Check sheet for the modelled part. Datum: model origin and axes. Units: mm. A direction names the side the tool comes from. Round coordinates to 2 decimals unless told otherwise and drop trailing zeros. Write each loop counter-clockwise with the first axis right and the second up, starting at its lowest first coordinate (ties: lowest second). Pieces come first, ordered by that corner, then holes. Notation, with made-up numbers: M -9.5,-39.75 L 2.5,-39.75 A19 ccw 2.5,-18.75 Z; hole C 52.25,17.25 d11. An arc over 180 degrees is marked long. Answer in a Markdown table with one row per item.
```python
from build123d import *

# Parameters (mm, degrees)
SKETCH1_W           = 45
SKETCH1_H           = 20
BOSS_EXTRUDE1_DEPTH = 1
SKETCH2_R           = 7.5
SKETCH2_R_2         = 6.5
BOSS_EXTRUDE2_DEPTH = 12
SKETCH3_R           = 6.5
BOSS_EXTRUDE3_DEPTH = 10


with BuildPart() as part:
    # Sketch1 → Boss-Extrude1 (new body)
    with BuildSketch(Plane.XY):
        with Locations((-3.47266881, 2.258842444)):
            Rectangle(SKETCH1_W, SKETCH1_H)
    extrude(amount=BOSS_EXTRUDE1_DEPTH)

    # Sketch2 → Boss-Extrude2 (add)
    with BuildSketch(Plane.XY):
        with Locations((-16.47266881, 2.258842444)):
            Circle(SKETCH2_R)
        with Locations((-16.47266881, 2.258842444)):
            Circle(SKETCH2_R_2, mode=Mode.SUBTRACT)
        with Locations((9.52733119, 2.258842444)):
            Circle(SKETCH2_R)
        with Locations((9.52733119, 2.258842444)):
            Circle(SKETCH2_R_2, mode=Mode.SUBTRACT)
    extrude(amount=-BOSS_EXTRUDE2_DEPTH)

    # Sketch3 → Boss-Extrude3 (add)
    with BuildSketch(Plane.XY):
        with Locations((9.52733119, 2.258842444)):
            Circle(SKETCH3_R)
        with Locations((-16.47266881, 2.258842444)):
            Circle(SKETCH3_R)
    extrude(amount=-BOSS_EXTRUDE3_DEPTH)


solid = part.part
```
1. Section check D-D, the plane z = -11. Record the cut outline in (x, y).
Found:
| item | result |
|---|---|
| outline | C -16.47,2.26 d15; C 9.53,2.26 d15; hole C -16.47,2.26 d13; hole C 9.53,2.26 d13 |
2. Section check B-B, the plane y = 6.75. Record the cut outline in (x, z), and give its area (3 significant figures).
Found:
| item | result |
|---|---|
| outline | M -25.97,0 L -22.48,0 L -22.48,-12 L -21.17,-12 L -21.17,-10 L -11.77,-10 L -11.77,-12 L -10.47,-12 L -10.47,0 L 3.52,0 L 3.52,-12 L 4.83,-12 L 4.83,-10 L 14.23,-10 L 14.23,-12 L 15.53,-12 L 15.53,0 L 19.03,0 L 19.03,1 L -25.97,1 Z |
| area | 296 mm2 |
3. Access from +Z, -Z, +X, -X, +Y, -Y to the whole of each face (thin tool, end or side, straight path). Record for faces 4 (the face through (-3.8, -7.741, 0.5)), 5 (the face through (9, 2, -10)).
Found:
| item | result |
|---|---|
| face 4 | +Z, -Z, +X, -X, -Y |
| face 5 | -Z |
4. Draft check along Y on faces 1 (the face through (4.737, 6.652, -10.986)), 2 (the face through (16.455, -0.614, -5.916)), 3 (the face through (-4, 2, 0)). Enter one of: +Y half, -Y half, draft (parallel to the pull), parting line (faces both ways), or undercut.
Found:
| item | result |
|---|---|
| face 1 | undercut |
| face 2 | parting line |
| face 3 | draft |
5. Scan lines: L1, parallel to X at y = 4.5, z = -10.25; L2, parallel to X at y = -1.5, z = -3.5; L3, parallel to Z at x = -3.5, y = 2.75. Record each from-to range of solid material in increasing order.
Found:
| item | result |
|---|---|
| L1 | x = -23.63 to -22.57, -10.37 to -9.32, 2.37 to 3.43, 15.63 to 16.68 |
| L2 | x = -22.96 to -9.98, 3.04 to 16.02 |
| L3 | z = 0 to 1 |
6. Section check C-C, the plane z = -6. Record the cut outline in (x, y).
Found:
| item | result |
|---|---|
| outline | C -16.47,2.26 d15; C 9.53,2.26 d15 |
7. Go/stop test with flat-tipped pins: pin 1 (3 mm diameter, centred on y = 9.5, z = -5.5, fed in from -X); pin 2 (5 mm diameter, centred on y = 7.5, z = -7, fed in from +X); pin 3 (4 mm diameter, centred on x = 9.5, y = 4.5, fed in from -Z). Record where each tip stops, or that it passes through.
Found:
| item | result |
|---|---|
| pin 1 | stops at x = -21.3 |
| pin 2 | stops at x = 16.51 |
| pin 3 | stops at z = -10 |
8. Section check A-A, the plane x = -14.5. Record the cut outline in (y, z), and give its area (3 significant figures).
Found:
| item | result |
|---|---|
| outline | M -7.74,0 L -4.98,0 L -4.98,-12 L -3.93,-12 L -3.93,-10 L 8.45,-10 L 8.45,-12 L 9.49,-12 L 9.49,0 L 12.26,0 L 12.26,1 L -7.74,1 Z |
| area | 169 mm2 |
